```python
from build123d import *

# Parameters (mm, degrees)
SKETCH1_W           = 41
SKETCH1_H           = 38
SKETCH1_R           = 1.55
SKETCH1_R_2         = 12
BOSS_EXTRUDE1_DEPTH = 5
SKETCH2_W           = 41
SKETCH2_H           = 4.5
BOSS_EXTRUDE2_DEPTH = 20
SKETCH3_R           = 2.05
BOSS_EXTRUDE3_DEPTH = 5
FILLET1_R           = 2


with BuildPart() as part:
    # Sketch1 → Boss-Extrude1 (new body)
    with BuildSketch(Plane.XY):
        Rectangle(SKETCH1_W, SKETCH1_H)
        with Locations((15.5, 15.5)):
            Circle(SKETCH1_R, mode=Mode.SUBTRACT)
        with Locations((-15.5, 15.5)):
            Circle(SKETCH1_R, mode=Mode.SUBTRACT)
        with Locations((15.5, -15.5)):
            Circle(SKETCH1_R, mode=Mode.SUBTRACT)
        with Locations((-15.5, -15.5)):
            Circle(SKETCH1_R, mode=Mode.SUBTRACT)
        Circle(SKETCH1_R_2, mode=Mode.SUBTRACT)
    extrude(amount=BOSS_EXTRUDE1_DEPTH)

    # Sketch2 → Boss-Extrude2 (add)
    with BuildSketch(Plane.XY.offset(5)):
        with Locations((0, 21.25)):
            Rectangle(SKETCH2_W, SKETCH2_H)
        with Locations((0, -21.25)):
            Rectangle(SKETCH2_W, SKETCH2_H)
    extrude(amount=-BOSS_EXTRUDE2_DEPTH)

    # Sketch3 → Boss-Extrude3 (add)
    # profile 1 of 2: a face of its own
    with BuildSketch(Plane(origin=(0, 0, -15), x_dir=(-1, 0, 0), z_dir=(0, 0, -1))):
        with BuildLine():
            Line((-20.5, 26.495282599), (-20.5, 23.5))
            Line((-20.5, 23.5), (20.5, 23.5))
            Line((20.5, 23.5), (20.5, 26.495282599))
            ThreePointArc((20.5, 26.495282599), (10.831851903, 31.700488708), (-7.9e-08, 33.5))
            ThreePointArc((-7.9e-08, 33.5), (-10.831851978, 31.700488683), (-20.5, 26.495282599))
        make_face()
        with Locations((-8.80698434, 27.105110714)):
            Circle(SKETCH3_R, mode=Mode.SUBTRACT)
        with Locations((8.80698434, 27.105110714)):
            Circle(SKETCH3_R, mode=Mode.SUBTRACT)
    # profile 2 of 2: a face of its own
    with BuildSketch(Plane(origin=(0, 0, -15), x_dir=(-1, 0, 0), z_dir=(0, 0, -1))):
        with BuildLine():
            Line((-20.5, -23.5), (-20.5, -26.495282599))
            ThreePointArc((-20.5, -26.495282599), (-10.831851978, -31.700488683), (-7.9e-08, -33.5))
            ThreePointArc((-7.9e-08, -33.5), (10.831851903, -31.700488708), (20.5, -26.495282599))
            Line((20.5, -26.495282599), (20.5, -23.5))
            Line((20.5, -23.5), (-20.5, -23.5))
        make_face()
        with Locations((-8.80698434, -27.105110714)):
            Circle(SKETCH3_R, mode=Mode.SUBTRACT)
        with Locations((8.80698434, -27.105110714)):
            Circle(SKETCH3_R, mode=Mode.SUBTRACT)
    extrude(amount=-BOSS_EXTRUDE3_DEPTH)

    # Fillet1
    fillet1_edges = [part.edges().sort_by_distance(p)[0] for p in [
        (20.5, 23.5, -2.5),
        (-20.5, 23.5, -2.5),
        (-20.5, -23.5, -2.5),
        (20.5, -23.5, -2.5),
    ]]
    fillet(fillet1_edges, radius=FILLET1_R)


solid = part.part
```
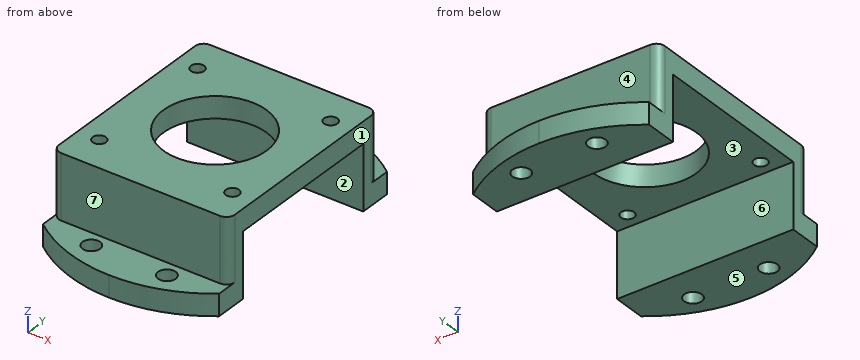
Input: part model. Units: mm. Frame: model coordinates. Face numbers are marked on the shaded views. A direction names the side the tool comes from. Give positions to 0.01 mm unless a question says otherwise; leave off trailing zeros. Order: outer loops, then holes, each group sorted by start corner. A loop starts at its lowest first (then second) coordinate and runs counter-clockwise, first axis right, second up. Notation, with made-up numbers: (5.5, -36) - (51.5, -36) arc R19 cw to (51.5, -31) - close; hole circle Ø10 at (-8, 55). An arc over 180 degrees is marked (long way). Use a Markdown table: item, result.
(1) Access query for the marked faces 5, 6 and 7. Directions: +Z, -Z, +X, -X, +Y, -Y. A direction counts if a zero-diameter tool reaches every point of the face in a straight line with its end or side. Return the directions, or none.
Computed values:
| item | result |
|---|---|
| face 5 | -Z, +X, -X, +Y, -Y |
| face 6 | -Z, +X, -X |
| face 7 | +Z, +X, -X, -Y |
(2) Line query: line 1 (Y direction, x = -15.5, z = 2.75); line 2 (Y direction, x = -3.5, z = -4.75); line 3 (Y direction, x = 10, z = -14). Output: solid intervals per line, ascending. Write a range as from..to.
Computed values:
| item | result |
|---|---|
| line 1 | y = -23.5..-17.05, -13.95..13.95, 17.05..23.5 |
| line 2 | y = -23.5..-19, 19..23.5 |
| line 3 | y = -31.97..-28.77, -25.44..-19, 19..25.44, 28.77..31.97 |
(3) Section query C-C (x = -16). Output: boundary loops of the cut face in (y, z).
Computed values:
| item | result |
|---|---|
| outline | (-29.43, -15) - (-19, -15) - (-19, 0) - (-16.97, 0) - (-16.97, 5) - (-23.5, 5) - (-23.5, -10) - (-29.43, -10) - close; (-14.03, 0) - (14.03, 0) - (14.03, 5) - (-14.03, 5) - close; (16.97, 0) - (19, 0) - (19, -15) - (29.43, -15) - (29.43, -10) - (23.5, -10) - (23.5, 5) - (16.97, 5) - close |
(4) Draft query along Y for the marked faces 1, 2, 3 and 4. Return one class per face: released by +Y, released by -Y, zero draft, split by the parting line, or undercut.
Computed values:
| item | result |
|---|---|
| face 1 | zero draft |
| face 2 | undercut |
| face 3 | undercut |
| face 4 | released by +Y |
(5) Pin query (flat end, axial travel): pin 1 (4 mm diameter, centred on x = 15.5, y = 15.5, fed in from -Z); pin 2 (6.5 mm diameter, centred on x = 8.81, y = -27.11, fed in from -Z); pin 3 (7.5 mm diameter, centred on x = -1, z = 0, fed in from -Y); pin 4 (2.5 mm diameter, centred on x = -15.5, y = -15.5, fed in from -Z). Return the tip coordinate at first contact, or that it passes through.
Computed values:
| item | result |
|---|---|
| pin 1 | stops at z = 0 |
| pin 2 | stops at z = -15 |
| pin 3 | stops at y = -23.5 |
| pin 4 | passes through |
(6) Section query D-D (z = -13.5). Output: boundary loops of the cut face in (x, y).
Computed values:
| item | result |
|---|---|
| outline | (-20.5, -26.5) arc R33.5 ccw to (20.5, -26.5) - (20.5, -19) - (-20.5, -19) - close; (-20.5, 19) - (20.5, 19) - (20.5, 26.5) arc R33.5 ccw to (-20.5, 26.5) - close; hole circle Ø4.1 at (-8.81, -27.11); hole circle Ø4.1 at (-8.81, 27.11); hole circle Ø4.1 at (8.81, -27.11); hole circle Ø4.1 at (8.81, 27.11) |
(7) Section query B-B (y = 15.5). Output: boundary loops of the cut face in (x, z), then the cut area to 3 significant figures.
Computed values:
| item | result |
|---|---|
| outline | (-20.5, 0) - (-17.05, 0) - (-17.05, 5) - (-20.5, 5) - close; (-13.95, 0) - (13.95, 0) - (13.95, 5) - (-13.95, 5) - close; (17.05, 0) - (20.5, 0) - (20.5, 5) - (17.05, 5) - close |
| area | 174 mm2 |
(8) Section query A-A (z = -6.5). Output: boundary loops of the cut face in (x, y), then the cut area to 3 significant figures.
Computed values:
| item | result |
|---|---|
| outline | (-20.5, -21.5) arc R2 ccw to (-18.5, -23.5) - (18.5, -23.5) arc R2 ccw to (20.5, -21.5) - (20.5, -19) - (-20.5, -19) - close; (-20.5, 19) - (20.5, 19) - (20.5, 21.5) arc R2 ccw to (18.5, 23.5) - (-18.5, 23.5) arc R2 ccw to (-20.5, 21.5) - close |
| area | 366 mm2 |
